Solid Edge part; units mm, degrees
sketch "Sketch1" plane through (0, 0, 0) normal (1, 0, 0) x (0, 1, 0)
  line L0 (10, 20) -> (10, 30)
  line L1 (0, 20) -> (10, 20)
sketch "Sketch2" plane through (0, 0, 0) normal (0, -1, 0) x (1, 0, 0)
  line L0 (0, 20) -> (-3, 20)
  line L1 (-3, 20) -> (-3, 19)
  line L2 (-3, 19) -> (-1.25, 19)
  line L3 (-1.25, 19) -> (-1.25, 0)
  line L4 (-1.25, 0) -> (0, 0)
  line L5 (0, 0) -> (0, 20)
sweep "ProtrusioneScorrimento_3" add profiles "Sketch2" path "Sketch1"
Can you work these out from the model? Positions are in its coordinate system, mm. A direction names the side the tool comes from. Give positions to 0.01 mm unless a question says otherwise; leave off trailing zeros. Order: outer loops, then holes, each group sorted by start corner. A loop starts at its lowest first (then second) coordinate and runs counter-clockwise, first axis right, second up. Notation, with made-up numbers: M 11,13.5 L 42,13.5 A34 ccw 42,43.5 Z; hole C -24.75,-27.5 d1. An arc over 180 degrees is marked long. Use one line per item in the form item = value.
Item 1: Thinking about a two-plate mould opening in Z: for faces 4 (the flat face through (-1, 5, 20)), 5 (the flat face through (-1, 15, 0)), 6 (the flat face through (-1, 0, 10)), which applies, pulls with the +Z half, pulls with the -Z half, needs draft (parallel to the pull), parting line crosses it, or undercut?
Values follow:
face_4 = pulls with the +Z half
face_5 = pulls with the -Z half
face_6 = needs draft
Item 2: If we section it at B-B, the plane z = 21.25: Write out the boundary of the cut face in (x, y), and give its area (4 significant figures).
Values follow:
outline = M -3,10 L 0,10 L 0,30 L -1.25,30 L -1.25,11 L -3,11 Z
area = 26.75 mm^2
Item 3: If we section it at A-A, the plane x = -0.8: Write out the boundary of the cut face in (y, z).
Values follow:
outline = M 0,0 L 30,0 L 30,30 L 10,30 L 10,20 L 0,20 Z
Item 4: Will these pins go through, and if not, where does the flat tip stop? pin 1 Ø0.9 at (x, y) = (-2, 4.5) entering from -Z; pin 2 Ø1 at (y, z) = (12, 4) entering from -X; pin 3 Ø0.9 at (x, y) = (-2, 3) entering from +Z.
Values follow:
pin_1 = 19
pin_2 = -1.25
pin_3 = 20
Item 5: If we section it at C-C, the plane y = 22: Write out the boundary of the cut face in (x, z), and give its area (3 significant figures).
Values follow:
outline = M -1.25,0 L 0,0 L 0,30 L -1.25,30 Z
area = 37.5 mm^2
Item 6: If I drill on line 1 along X through (y, z) = (21, 7.5); line 2 along Z through (x, y) = (-1.7, 7); line 3 along Z through (x, y) = (-0.45, 2), over which ranges is the centre line in solid material (lowest first)? Write a range as [from, to].
Values follow:
line_1 = [-1.25, 0]
line_2 = [19, 20]
line_3 = [0, 20]
Item 7: For faces 1 (the flat face through (-2, 6, 19)), 2 (the flat face through (-2, 11, 25)), 3 (the flat face through (-1, 10, 25)), which set-ups out of +Z, -Z, +X, -X, +Y, -Y let a thin tool reach every point of the face, with its end or its side?
Values follow:
face_1 = -Z, -X, +Y, -Y
face_2 = +Z, -Z, -X, +Y
face_3 = +Z, +X, -X, -Y
